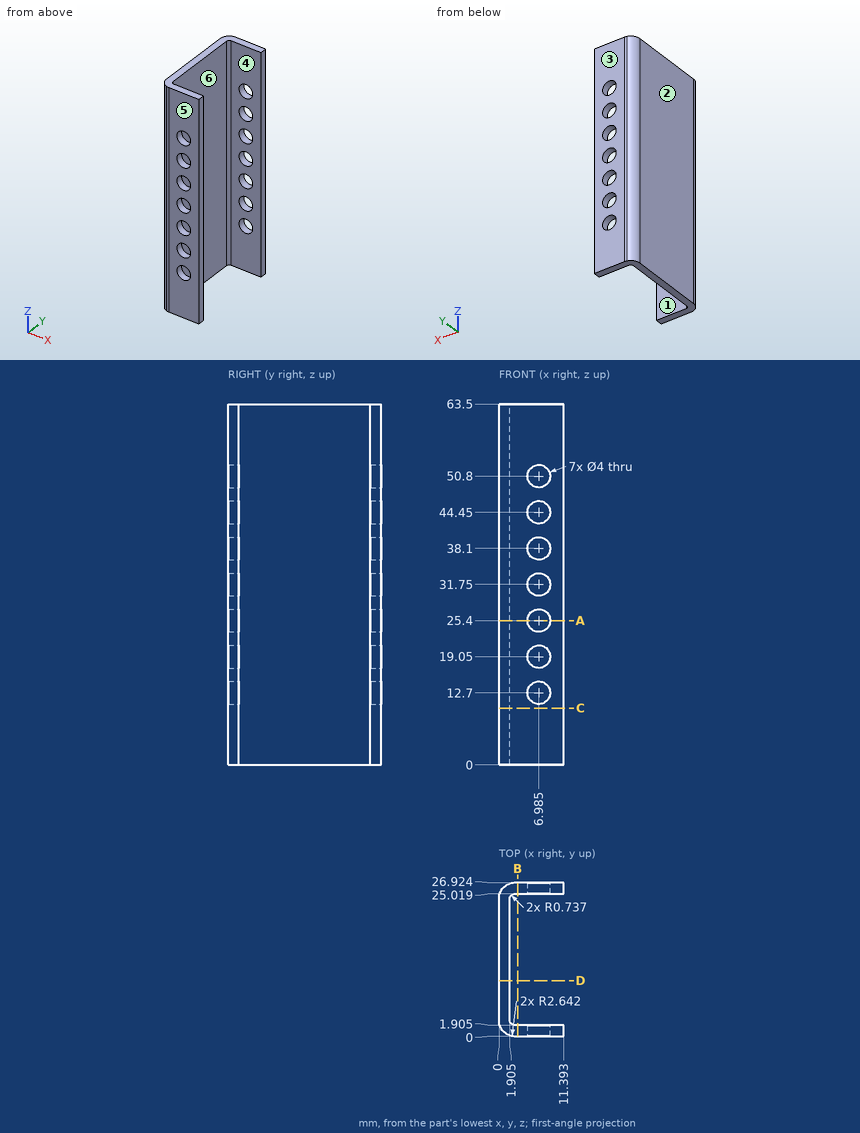
Geometry: see drawing. Coordinates: mm, zero at the bounding-box minimum. A direction names the side the tool comes from. Coordinates: 2 decimals unless noted, no trailing zeros. Order: outer loops, then holes, each group sorted by start corner. A loop starts at its lowest first (then second) coordinate and runs counter-clockwise, first axis right, second up. Notation, with made-up numbers: (47, 42.25) - (53, 42.25) arc R30 ccw to (53, 73.25) - close; hole circle Ø9 at (-7.75, -35). An arc over 180 degrees is marked (long way). Write each question's results on one line, items separated by ' | '.
1) Section C-C, the plane z = 10. Return loops of the section in (x, y) (1 decimal).
Results list:
outline: (0, 2.6) arc R2.6 ccw to (2.6, 0) - (11.4, 0) - (11.4, 1.9) - (2.6, 1.9) arc R0.7 cw to (1.9, 2.6) - (1.9, 24.3) arc R0.7 cw to (2.6, 25) - (11.4, 25) - (11.4, 26.9) - (2.6, 26.9) arc R2.6 ccw to (0, 24.3) - close
2) Section A-A, the plane z = 25.4. Return loops of the section in (x, y) (1 decimal).
Results list:
outline: (0, 2.6) arc R2.6 ccw to (2.6, 0) - (5, 0) - (5, 1.9) - (2.6, 1.9) arc R0.7 cw to (1.9, 2.6) - (1.9, 24.3) arc R0.7 cw to (2.6, 25) - (5, 25) - (5, 26.9) - (2.6, 26.9) arc R2.6 ccw to (0, 24.3) - close; (9, 0) - (11.4, 0) - (11.4, 1.9) - (9, 1.9) - close; (9, 25) - (11.4, 25) - (11.4, 26.9) - (9, 26.9) - close
3) Line query: line 1 (Y direction, x = 10.25, z = 60) (1 decimal); line 2 (X direction, y = 5, z = 14) (1 decimal); line 3 (Y direction, x = 1.25, z = 38.5) (1 decimal). Output: solid intervals per line, ascending. Write a range as from..to.
Results list:
line 1: 0..1.9, 25..26.9 | line 2: 0..1.9 | line 3: 0.4..26.5
4) Section D-D, the plane y = 9.75. Return loops of the section in (x, z) (1 decimal).
Results list:
outline: (0, 0) - (1.9, 0) - (1.9, 63.5) - (0, 63.5) - close
5) Pull-direction query (Y, two-part tool) for the marked faces 1, 2, 3 and 4; classes: pulls with the +Y half, pulls with the -Y half, needs draft (parallel to the pull), parting line crosses it, or undercut.
Results list:
face 1: undercut | face 2: needs draft | face 3: pulls with the +Y half | face 4: undercut
6) Pin query (flat end, axial travel): pin 1 (2.5 mm diameter, centred on x = 6.985, z = 44.45, fed in from -Y); pin 2 (4.5 mm diameter, centred on x = 6.985, z = 50.8, fed in from -Y); pin 3 (1.5 mm diameter, centred on y = 18.5, z = 42.5, fed in from +X) (3 decimals). Return the tip coordinate at first contact, or that it passes through.
Results list:
pin 1: through | pin 2: y = 0 | pin 3: x = 1.905
7) Set-up query: the marked faces 5 and 6. Return all of +Z, -Z, +X, -X, +Y, -Y with unobstructed straight access to the full face (end or side cutting, diameter ignored); none if empty.
Results list:
face 5: +Z, -Z, +X, -X, -Y | face 6: +Z, -Z, +X
8) Section B-B, the plane x = 3.25. Return loops of the section in (y, z) (1 decimal).
Results list:
outline: (0, 0) - (1.9, 0) - (1.9, 63.5) - (0, 63.5) - close; (25, 0) - (26.9, 0) - (26.9, 63.5) - (25, 63.5) - close
